from build123d import *

# Parameters (mm, degrees)
BOSS_EXTRUDE1_START     = -12.827
BOSS_EXTRUDE1_DEPTH     = 3.175
M5_CLEARANCE_HOLE1_D    = 5.8
F_1_4_CLEARANCE_HOLE1_D = 7.14248
FILLET1_R               = 3.175


with BuildPart() as part:
    # Sketch1 → Boss-Extrude1 (new body)
    with BuildSketch(Plane(origin=(0, 144.904574554, 0), x_dir=(1, 0, 0), z_dir=(0, 1, 0)).offset(BOSS_EXTRUDE1_START)):
        with BuildLine():
            Line((-78.14945, -1144.867512521), (-37.25545, -1144.867512521))
            ThreePointArc((-37.25545, -1144.867512521), (-33.208181466, -1146.564417216), (-31.581293209, -1150.640334625))
            Line((-31.581293209, -1150.640334625), (-33.994293209, -1290.605977985))
            ThreePointArc((-33.994293209, -1290.605977985), (-35.690354742, -1294.555424368), (-39.66845, -1296.183155787))
            Line((-39.66845, -1296.183155787), (-75.73645, -1296.183155787))
            ThreePointArc((-75.73645, -1296.183155787), (-79.714545258, -1294.555424368), (-81.410606791, -1290.605977985))
            Line((-81.410606791, -1290.605977985), (-81.469319904, -1287.200334154))
            Line((-81.469319904, -1287.200334154), (-114.966812484, -1287.200334154))
            ThreePointArc((-114.966812484, -1287.200334154), (-121.702004575, -1284.410526245), (-124.491812484, -1277.675334154))
            Line((-124.491812484, -1277.675334154), (-124.491812484, -1220.525334154))
            Line((-124.491812484, -1220.525334154), (-124.491812484, -1163.375334154))
            ThreePointArc((-124.491812484, -1163.375334154), (-121.702004575, -1156.640142063), (-114.966812484, -1153.850334154))
            Line((-114.966812484, -1153.850334154), (-83.768266576, -1153.850334154))
            Line((-83.768266576, -1153.850334154), (-83.823606791, -1150.640334625))
            ThreePointArc((-83.823606791, -1150.640334625), (-82.196718534, -1146.564417216), (-78.14945, -1144.867512521))
        make_face()
    extrude(amount=-BOSS_EXTRUDE1_DEPTH)

    # M5 Clearance Hole1 (through all)
    with Locations(Plane(origin=(0, 128.902574554, 0), x_dir=(-1, 0, 0), z_dir=(0, -1, 0))):
        with Locations((39.66845, -1290.508155834), (75.73645, -1290.508155834), (37.25545, -1150.542512474), (78.14945, -1150.542512474)):
            Hole(M5_CLEARANCE_HOLE1_D / 2)

    # 1/4 Clearance Hole1 (through all)
    with Locations(Plane(origin=(0, 132.077574554, 0), x_dir=(1, 0, 0), z_dir=(0, 1, 0))):
        with Locations((-0.438087516, -1163.375334154), (-0.438087516, -1220.525334154), (-0.438087516, -1277.675334154), (-114.966812484, -1163.375334154), (-114.966812484, -1220.525334154), (-114.966812484, -1277.675334154)):
            Hole(F_1_4_CLEARANCE_HOLE1_D / 2)

    # Fillet1
    fillet1_edges = [part.edges().sort_by_distance(p)[0] for p in [
        (-81.469319904, 130.490074554, 1287.200334154),
        (-83.768266576, 130.490074554, 1153.850334154),
    ]]
    fillet(fillet1_edges, radius=FILLET1_R)


solid = part.part
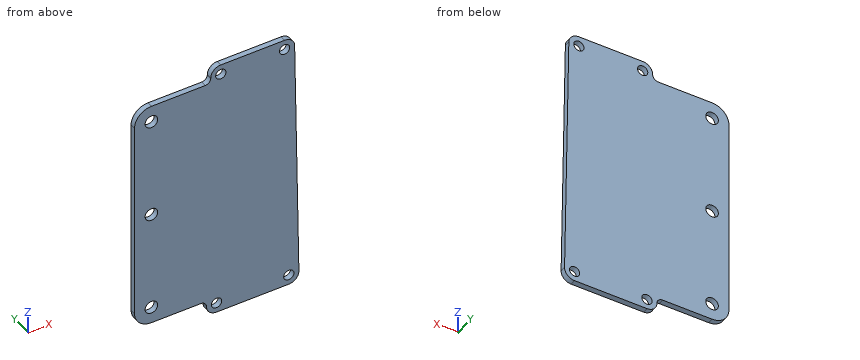
Here's how the part is built. I have some questions about the finished solid (model axes, mm). Coordinates: 2 decimals unless noted, no trailing zeros. Write each loop counter-clockwise with the first axis right and the second up, starting at its lowest first coordinate (ties: lowest second). Pieces come first, ordered by that corner, then holes. Notation, with made-up numbers: (70, -29.5) - (95, -29.5) arc R25 ccw to (95, 7.5) - close; hole circle Ø7 at (-7.5, 40.25). An arc over 180 degrees is marked (long way). Use one line per item in the form item = value.
1) I need wall thicknesses on line 1 (Z direction, x = -113, y = 130.55); line 2 (Z direction, x = -116.5, y = 131.3); line 3 (Z direction, x = -76, y = 129.25). Which ranges of each line are inside material? Lowest first, please.
Solved:
line_1 = 1153.85 to 1160.39, 1166.36 to 1217.54, 1223.51 to 1274.69, 1280.66 to 1287.2
line_2 = 1153.97 to 1160.15, 1166.6 to 1217.3, 1223.75 to 1274.45, 1280.9 to 1287.08
line_3 = 1144.87 to 1148.6, 1152.49 to 1287.62, 1293.4 to 1296.18
2) Suppose I cut it at C-C, the plane z = 1272.5. Write out the boundary of the cut face in (x, y), plus the area to 3 significant figures.
Solved:
outline = (-124.49, 128.9) - (-33.68, 128.9) - (-33.68, 132.08) - (-124.49, 132.08) - close
area = 288 mm2
3) Suppose I cut it at B-B, the plane y = 131. Give the number of separate pieces and of enclosed holes in the cut face, plus the area to 3 significant figures.
Solved:
separate_pieces = 1
enclosed_holes = 7
area = 12,800 mm2
4) Suppose I cut it at A-A, the plane x = -108. Write out the boundary of the cut face in (y, z).
Solved:
outline = (128.9, 1153.85) - (132.08, 1153.85) - (132.08, 1287.2) - (128.9, 1287.2) - close
5) I'm going to push flat-ended pins straight in: P1, Ø1, axis at x = -101, y = 130.5, coming from the -Z side; P2, Ø1.5, axis at x = -90, y = 131, coming from the +Z side. Where does each tip first touch, or does it pass through?
Solved:
P1 = 1153.85
P2 = 1287.2
